Job drawing, mm, ordinate dimensions from the low corner. One solid piece. A direction names the side the tool comes from. Give positions to 0.01 mm unless a question says otherwise; leave off trailing zeros. Loops run counter-clockwise (first coordinate to the right, second up) from the corner with the lowest first, then second, coordinate; pieces in that order, holes last. Notation, with made-up numbers: M 56.25,76.5 L 78.25,76.5 A18 cw 78.25,110.5 Z; hole C 9.25,76.25 d7. An arc over 180 degrees is marked long. Put each result on its own line as item: value.
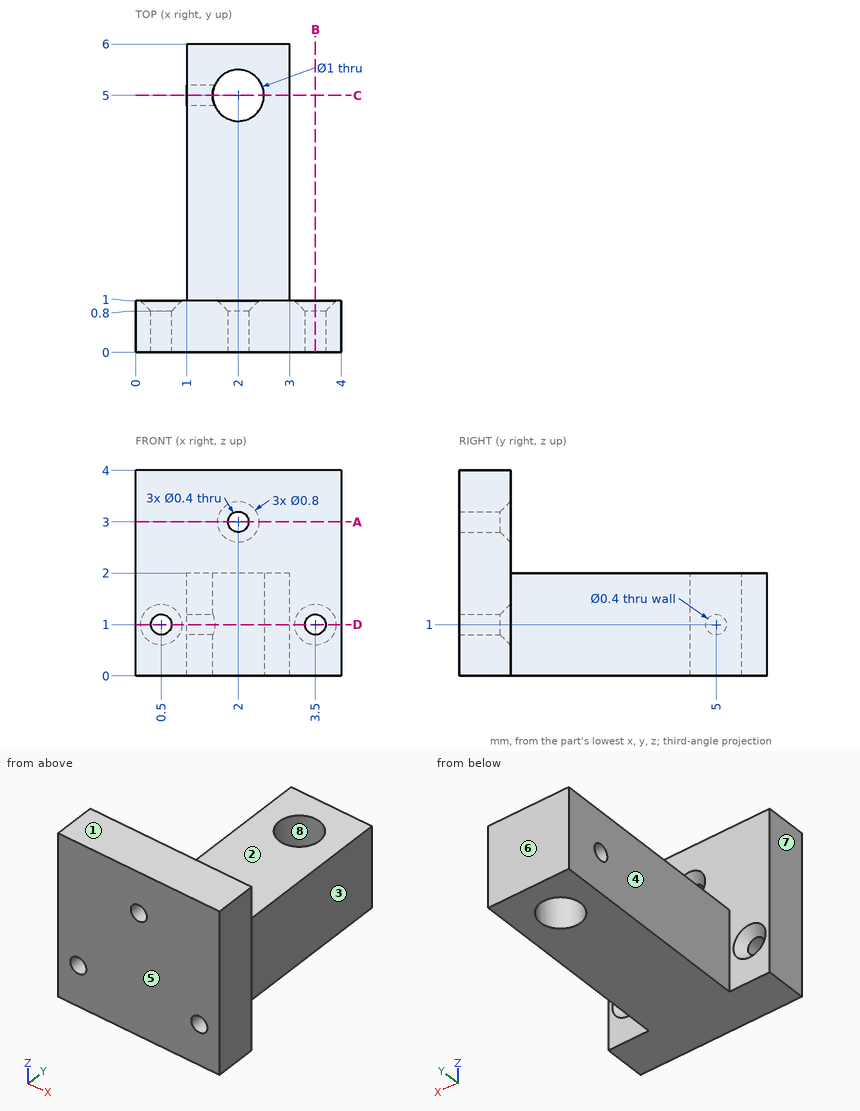
Q1. Slice it at C-C (y = 5). List the corners of the cut face in (x, z).
Here are the results:
outline: M 1,0 L 1.5,0 L 1.5,0.8 L 1,0.8 Z; M 1,1.2 L 1.5,1.2 L 1.5,2 L 1,2 Z; M 2.5,0 L 3,0 L 3,2 L 2.5,2 Z
Q2. Slice it at A-A (z = 3). List the corners of the cut face in (x, y).
Here are the results:
outline: M 0,0 L 1.8,0 L 1.8,0.8 L 1.6,1 L 0,1 Z; M 2.2,0 L 4,0 L 4,1 L 2.4,1 L 2.2,0.8 Z
Q3. Drop flat-ended pins along their axis: pin 1 Ø0.6 at (y, z) = (2.5, 1) entering from -X; pin 2 Ø0.6 at (y, z) = (2.5, 1) entering from +X; pin 3 Ø1.2 at (x, z) = (2, 2.5) entering from +Y; pin 4 Ø1.6 at (x, y) = (1.5, 2.5) entering from +Z. Give the stop position or say it passes through.
Here are the results:
pin 1: x = 1
pin 2: x = 3
pin 3: y = 6
pin 4: z = 2
Q4. Tool access for the marked faces 1, 2, 3 and 4: list every direction of +Z, -Z, +X, -X, +Y, -Y with a clear straight run to the whole face (end or side of a thin tool).
Here are the results:
face 1: +Z, +X, -X, +Y, -Y
face 2: +Z, +X, -X, +Y
face 3: +Z, -Z, +X, +Y
face 4: +Z, -Z, -X, +Y
Q5. Slice it at D-D (z = 1). List the corners of the cut face in (x, y).
Here are the results:
outline: M 0,0 L 0.3,0 L 0.3,0.8 L 0.1,1 L 0,1 Z; M 0.7,0 L 3.3,0 L 3.3,0.8 L 3.1,1 L 3,1 L 3,6 L 1,6 L 1,5.2 L 1.54,5.2 A0.5 cw long 1.54,4.8 L 1,4.8 L 1,1 L 0.9,1 L 0.7,0.8 Z; M 3.7,0 L 4,0 L 4,1 L 3.9,1 L 3.7,0.8 Z
Q6. Slice it at B-B (x = 3.5). List the corners of the cut face in (y, z), and give its area (3 significant figures).
Here are the results:
outline: M 0,0 L 1,0 L 1,0.6 L 0.8,0.8 L 0,0.8 Z; M 0,1.2 L 0.8,1.2 L 1,1.4 L 1,4 L 0,4 Z
area: 3.56 mm²
Q7. Probe line 1 (Z direction, x = 1.4, y = 5); line 2 (Y direction, x = 2.05, z = 0.25); line 3 (Z direction, x = 0.5, y = 0.5). List the from-to ranges inside material, lowest first. Write a range as from..to.
Here are the results:
line 1: 0..0.8, 1.2..2
line 2: 0..4.5, 5.5..6
line 3: 0..0.8, 1.2..4
Q8. Mould opens along Y. For the marked faces 5, 6, 7 and 8 say: pulls with the +Y half, pulls with the -Y half, needs draft (parallel to the pull), parting line crosses it, or undercut.
Here are the results:
face 5: pulls with the -Y half
face 6: pulls with the +Y half
face 7: needs draft
face 8: undercut
